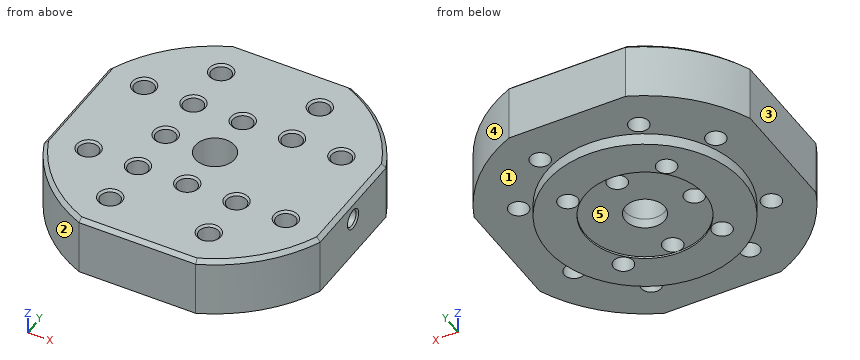
from build123d import *

# Parameters (mm, degrees)
SKIZZE1_R                       = 5
AUFSATZ_LINEAR_AUSTRAGEN1_DEPTH = 15
SKIZZE4_R                       = 24.75
AUFSATZ_LINEAR_AUSTRAGEN2_DEPTH = 3
SKIZZE2_R                       = 2.5
SCHNITT_LINEAR_AUSTRAGEN1_DEPTH = 20
M6_GEWINDEBOHRUNG1_D            = 5
M6_GEWINDEBOHRUNG1_DEPTH        = 10
M6_GEWINDEBOHRUNG1_CSINK_D      = 6.05
M6_GEWINDEBOHRUNG1_CSINK_ANGLE  = 90
M6_GEWINDEBOHRUNG1_TIP          = 1.502151548
SCHNITT_LINEAR_START            = -13.25
SKIZZE5_R                       = 5
SCHNITT_LINEAR_AUSTRAGEN2_DEPTH = 13.25
SKIZZE6_R                       = 60.631452858
SKIZZE6_R_2                     = 38
SCHNITT_LINEAR_AUSTRAGEN3_DEPTH = 17
FASE1_SIZE                      = 1
SKIZZE7_R                       = 2
SCHNITT_LINEAR_AUSTRAGEN4_DEPTH = 38
M5_GEWINDEBOHRUNG1_D            = 4.2
M5_GEWINDEBOHRUNG1_DEPTH        = 34
M5_GEWINDEBOHRUNG1_CSINK_D      = 5.05
M5_GEWINDEBOHRUNG1_CSINK_ANGLE  = 90
M5_GEWINDEBOHRUNG1_TIP          = 1.2618073
SKIZZE10_R                      = 15.05
SCHNITT_LINEAR_AUSTRAGEN5_DEPTH = 0.5


with BuildPart() as part:
    # Skizze1 → Aufsatz-Linear austragen1 (new body)
    with BuildSketch(Plane.XY):
        with BuildLine():
            Line((-36.910459775, 30.503472222), (29.089540225, 30.503472222))
            ThreePointArc((29.089540225, 30.503472222), (30.503753788, 29.917685785), (31.089540225, 28.503472222))
            Line((31.089540225, 28.503472222), (31.089540225, -37.496527778))
            ThreePointArc((31.089540225, -37.496527778), (30.503753788, -38.91074134), (29.089540225, -39.496527778))
            Line((29.089540225, -39.496527778), (-36.910459775, -39.496527778))
            ThreePointArc((-36.910459775, -39.496527778), (-38.324673337, -38.91074134), (-38.910459775, -37.496527778))
            Line((-38.910459775, -37.496527778), (-38.910459775, 28.503472222))
            ThreePointArc((-38.910459775, 28.503472222), (-38.324673337, 29.917685785), (-36.910459775, 30.503472222))
        make_face()
        with Locations((-3.910459775, -4.496527778)):
            Circle(SKIZZE1_R, mode=Mode.SUBTRACT)
    extrude(amount=AUFSATZ_LINEAR_AUSTRAGEN1_DEPTH)

    # Skizze4 → Aufsatz-Linear austragen2 (add)
    with BuildSketch(Plane(origin=(0, 0, 0), x_dir=(-1, 0, 0), z_dir=(0, 0, -1))):
        with Locations((3.910459775, -4.496527778)):
            Circle(SKIZZE4_R)
    extrude(amount=AUFSATZ_LINEAR_AUSTRAGEN2_DEPTH)

    # Skizze2 → Schnitt-Linear austragen1 (cut)
    with BuildSketch(Plane.XY.offset(15)):
        with Locations((-16.410459775, 20.503472222)):
            Circle(SKIZZE2_R)
        with Locations((8.589540225, 20.503472222)):
            Circle(SKIZZE2_R)
        with Locations((-16.410459775, 8.003472222)):
            Circle(SKIZZE2_R)
        with Locations((-3.910459775, 8.003472222)):
            Circle(SKIZZE2_R)
        with Locations((8.589540225, 8.003472222)):
            Circle(SKIZZE2_R)
        with Locations((21.089540225, 8.003472222)):
            Circle(SKIZZE2_R)
        with Locations((-16.410459775, -4.496527778)):
            Circle(SKIZZE2_R)
        with Locations((-16.410459775, -16.996527778)):
            Circle(SKIZZE2_R)
        with Locations((-3.910459775, -16.996527778)):
            Circle(SKIZZE2_R)
        with Locations((8.589540225, -16.996527778)):
            Circle(SKIZZE2_R)
        with Locations((21.089540225, -16.996527778)):
            Circle(SKIZZE2_R)
        with Locations((-16.410459775, -29.496527778)):
            Circle(SKIZZE2_R)
        with Locations((8.589540225, -29.496527778)):
            Circle(SKIZZE2_R)
        with Locations((-28.910459775, 8.003472222)):
            Circle(SKIZZE2_R)
        with Locations((-28.910459775, -16.996527778)):
            Circle(SKIZZE2_R)
    extrude(amount=-SCHNITT_LINEAR_AUSTRAGEN1_DEPTH, mode=Mode.SUBTRACT)

    # M6 Gewindebohrung1
    with Locations(Plane(origin=(-16.410459775, 20.503472222, 15), x_dir=(1, 0, 0), z_dir=(0, 0, 1))):
        with Locations((0, 0), (25, 0), (37.5, -12.5), (25, -12.5), (12.5, -12.5), (0, -12.5), (-12.5, -12.5), (0, -25), (37.5, -37.5), (25, -37.5), (12.5, -37.5), (0, -37.5), (-12.5, -37.5), (0, -50), (25, -50)):
            CounterSinkHole(M6_GEWINDEBOHRUNG1_D / 2, M6_GEWINDEBOHRUNG1_CSINK_D / 2, depth=M6_GEWINDEBOHRUNG1_DEPTH, counter_sink_angle=M6_GEWINDEBOHRUNG1_CSINK_ANGLE)
            with Locations((0, 0, -(M6_GEWINDEBOHRUNG1_DEPTH + M6_GEWINDEBOHRUNG1_TIP / 2))):  # 118° drill point
                Cone(0, M6_GEWINDEBOHRUNG1_D / 2, M6_GEWINDEBOHRUNG1_TIP, mode=Mode.SUBTRACT)

    # Skizze5 → Schnitt-Linear austragen2 (cut)
    with BuildSketch(Plane.XY.offset(SCHNITT_LINEAR_START)):
        with Locations(Location((-3.910459775, -4.496527778, 0), (0, 0, 180))):
            Circle(SKIZZE5_R)
    extrude(amount=SCHNITT_LINEAR_AUSTRAGEN2_DEPTH, mode=Mode.SUBTRACT)

    # Skizze6 → Schnitt-Linear austragen3 (cut)
    with BuildSketch(Plane.XY.offset(15)):
        with Locations((-3.910459775, -4.496527778)):
            Circle(SKIZZE6_R)
        with Locations((-3.910459775, -4.496527778)):
            Circle(SKIZZE6_R_2, mode=Mode.SUBTRACT)
    extrude(amount=-SCHNITT_LINEAR_AUSTRAGEN3_DEPTH, mode=Mode.SUBTRACT)

    # Fase1
    fase1_edges = [part.edges().sort_by_distance(p)[0] for p in [
        (-38.910459775, -4.496527778, 15),
        (-3.910459775, 30.503472222, 15),
        (31.089540225, -4.496527778, 15),
        (-3.910459775, -39.496527778, 15),
        (22.95959791, -31.366585463, 15),
        (22.95959791, 22.373529907, 15),
        (-30.78051746, 22.373529907, 15),
        (-30.78051746, -31.366585463, 15),
    ]]
    chamfer(fase1_edges, length=FASE1_SIZE)

    # Skizze7 → Schnitt-Linear austragen4 (cut)
    with BuildSketch(Plane(origin=(31.089540225, 0, 0), x_dir=(0, 0, -1), z_dir=(1, 0, 0))):
        with Locations(Location((-10, -4.496527778, 0), (0, 0, 90))):
            Circle(SKIZZE7_R)
    extrude(amount=-SCHNITT_LINEAR_AUSTRAGEN4_DEPTH, mode=Mode.SUBTRACT)

    # M5 Gewindebohrung1
    with Locations(Plane(origin=(31.089540225, -4.496527778, 10), x_dir=(0, 1, 0), z_dir=(1, 0, 0))):
        with Locations((0, 0)):
            CounterSinkHole(M5_GEWINDEBOHRUNG1_D / 2, M5_GEWINDEBOHRUNG1_CSINK_D / 2, depth=M5_GEWINDEBOHRUNG1_DEPTH, counter_sink_angle=M5_GEWINDEBOHRUNG1_CSINK_ANGLE)
            with Locations((0, 0, -(M5_GEWINDEBOHRUNG1_DEPTH + M5_GEWINDEBOHRUNG1_TIP / 2))):  # 118° drill point
                Cone(0, M5_GEWINDEBOHRUNG1_D / 2, M5_GEWINDEBOHRUNG1_TIP, mode=Mode.SUBTRACT)

    # Skizze10 → Schnitt-Linear austragen5 (cut)
    with BuildSketch(Plane(origin=(0, 0, -3), x_dir=(-1, 0, 0), z_dir=(0, 0, -1))):
        with Locations((3.910459775, -4.496527778)):
            Circle(SKIZZE10_R)
    extrude(amount=-SCHNITT_LINEAR_AUSTRAGEN5_DEPTH, mode=Mode.SUBTRACT)


solid = part.part
Geometry: final body of the model. Coordinates: model frame, mm. Face numbers are marked on the shaded views. A direction names the side the tool comes from. Give positions to 0.01 mm unless a question says otherwise; leave off trailing zeros. Write each loop counter-clockwise with the first axis right and the second up, starting at its lowest first coordinate (ties: lowest second). Pieces come first, ordered by that corner, then holes. Notation, with made-up numbers: (21, -20.5) - (34, -20.5) arc R34 ccw to (34, 12.5) - close; hole circle Ø7 at (-11.75, 36.25). An arc over 180 degrees is marked (long way). Return JSON: item names as keys, results as strings. Group by question number.
1) Set-up query: the marked faces 1 and 2. Return all of +Z, -Z, +X, -X, +Y, -Y with unobstructed straight access to the full face (end or side cutting, diameter ignored); none if empty.
2) Mould query, pull axis X, two halves, no side actions, for the marked faces 3, 4 and 5. Classes: released by +X, released by -X, zero draft, split by the parting line, or undercut.
3) First-contact query: P1, Ø8, axis at x = 21.09, y = 8, coming from the -Z side; P2, Ø3.5, axis at y = -4.5, z = 10, coming from the +X side; P3, Ø11.5, axis at x = -3.91, y = -4.5, coming from the -Z side; P4, Ø5, axis at x = -31.5, z = 4.5, coming from the +Y side. Flat tips, straight axial feed; report the tip coordinate or a pass-through.
4) Section B-B on x = 4.5. Return the cut outline in (y, z), plus the area to 3 significant figures.
5) Section A-A on z = 10. State how many separate pieces and enclosed holes the cut face has, plus the area to 3 significant figures.
6) Line query: line 1 (X direction, y = -4.5, z = 12.75); line 2 (X direction, y = -31, z = 11.75); line 3 (Y direction, x = -16, z = 0.5). Output: solid intervals per line, ascending.
7) Section C-C on y = 3. Return the cut outline in (x, z), plus the area to 3 significant figures.
Filled in:
{
 "1": {"face 1": "-Z", "face 2": "+Z, -Z, -X, -Y"},
 "2": {"face 3": "released by -X", "face 4": "released by +X", "face 5": "undercut"},
 "3": {"P1": "stops at z = -3", "P2": "stops at x = -8.59", "P3": "stops at z = -2.5", "P4": "stops at y = 24.04"},
 "4": {"outline": "(-39.5, 0) - (-27.77, 0) - (-27.77, -3) - (-16.98, -3) - (-16.98, -2.5) - (7.98, -2.5) - (7.98, -3) - (18.78, -3) - (18.78, 0) - (30.5, 0) - (30.5, 14) - (29.5, 15) - (-38.5, 15) - (-39.5, 14) - close; hole circle Ø4.2 at (-4.5, 10)", "area": "1,160 mm^2"},
 "5": {"separate pieces": "1", "enclosed holes": "15", "area": "3,800 mm^2"},
 "6": {"line 1": "x = -38.91 to -18.91, -13.91 to -8.91, 1.09 to 31.09", "line 2": "x = -31.14 to -18.41, -14.41 to 6.59, 10.59 to 23.32", "line 3": "y = -39.5 to -31.96, -27.03 to -19.46, -14.53 to -6.96, -2.03 to 5.54, 10.47 to 18.04, 22.97 to 30.5"},
 "7": {"outline": "(-38.91, 0) - (-27.5, 0) - (-27.5, -3) - (-16.96, -3) - (-16.96, -2.5) - (9.14, -2.5) - (9.14, -3) - (19.68, -3) - (19.68, 0) - (31.09, 0) - (31.09, 14) - (30.09, 15) - (-37.91, 15) - (-38.91, 14) - close", "area": "1,180 mm^2"}
}
